from build123d import *

# Parameters (mm, degrees)
F0_W     = 25.4
F0_H     = 50.8
F0_W_2   = 19.05
F0_H_2   = 44.45
F1_DEPTH = 228.6
F2_W     = 25.4
F2_H     = 457.2
F2_R     = 2.5527
F3_DEPTH = 50.801


with BuildPart() as f1:
    # F0 (on Front) → F1 (new body, symmetric)
    with BuildSketch(Plane.XZ):
        Rectangle(F0_W, F0_H)
        Rectangle(F0_W_2, F0_H_2, mode=Mode.SUBTRACT)
    extrude(amount=F1_DEPTH, both=True)

    # F2 (on face) → F3 (intersect, through all)
    with BuildSketch(Plane.XY.offset(25.4)):
        Rectangle(F2_W, F2_H)
        with Locations((-1.224507, -215.9)):
            Circle(F2_R, mode=Mode.SUBTRACT)
        with Locations((-1.224507, -203.2)):
            Circle(F2_R, mode=Mode.SUBTRACT)
        with Locations((-1.224507, -190.5)):
            Circle(F2_R, mode=Mode.SUBTRACT)
        with Locations((-1.224507, -177.8)):
            Circle(F2_R, mode=Mode.SUBTRACT)
        with Locations((-1.224507, -165.1)):
            Circle(F2_R, mode=Mode.SUBTRACT)
        with Locations((-1.224507, -152.4)):
            Circle(F2_R, mode=Mode.SUBTRACT)
        with Locations((-1.224507, -139.7)):
            Circle(F2_R, mode=Mode.SUBTRACT)
        with Locations((-1.224507, -127)):
            Circle(F2_R, mode=Mode.SUBTRACT)
        with Locations((-1.224507, -114.3)):
            Circle(F2_R, mode=Mode.SUBTRACT)
        with Locations((-1.224507, -101.6)):
            Circle(F2_R, mode=Mode.SUBTRACT)
        with Locations((-1.224507, -88.9)):
            Circle(F2_R, mode=Mode.SUBTRACT)
        with Locations((-1.224507, -76.2)):
            Circle(F2_R, mode=Mode.SUBTRACT)
        with Locations((-1.224507, -63.5)):
            Circle(F2_R, mode=Mode.SUBTRACT)
        with Locations((-1.224507, -50.8)):
            Circle(F2_R, mode=Mode.SUBTRACT)
        with Locations((-1.224507, -38.1)):
            Circle(F2_R, mode=Mode.SUBTRACT)
        with Locations((-1.224507, -25.4)):
            Circle(F2_R, mode=Mode.SUBTRACT)
        with Locations((-1.224507, -12.7)):
            Circle(F2_R, mode=Mode.SUBTRACT)
        with Locations((-1.224507, 0)):
            Circle(F2_R, mode=Mode.SUBTRACT)
        with Locations((-1.224507, 12.7)):
            Circle(F2_R, mode=Mode.SUBTRACT)
        with Locations((-1.224507, 25.4)):
            Circle(F2_R, mode=Mode.SUBTRACT)
        with Locations((-1.224507, 38.1)):
            Circle(F2_R, mode=Mode.SUBTRACT)
        with Locations((-1.224507, 50.8)):
            Circle(F2_R, mode=Mode.SUBTRACT)
        with Locations((-1.224507, 63.5)):
            Circle(F2_R, mode=Mode.SUBTRACT)
        with Locations((-1.224507, 76.2)):
            Circle(F2_R, mode=Mode.SUBTRACT)
        with Locations((-1.224507, 88.9)):
            Circle(F2_R, mode=Mode.SUBTRACT)
        with Locations((-1.224507, 101.6)):
            Circle(F2_R, mode=Mode.SUBTRACT)
        with Locations((-1.224507, 114.3)):
            Circle(F2_R, mode=Mode.SUBTRACT)
        with Locations((-1.224507, 127)):
            Circle(F2_R, mode=Mode.SUBTRACT)
        with Locations((-1.224507, 139.7)):
            Circle(F2_R, mode=Mode.SUBTRACT)
        with Locations((-1.224507, 152.4)):
            Circle(F2_R, mode=Mode.SUBTRACT)
        with Locations((-1.224507, 165.1)):
            Circle(F2_R, mode=Mode.SUBTRACT)
        with Locations((-1.224507, 177.8)):
            Circle(F2_R, mode=Mode.SUBTRACT)
        with Locations((-1.224507, 190.5)):
            Circle(F2_R, mode=Mode.SUBTRACT)
        with Locations((-1.224507, 203.2)):
            Circle(F2_R, mode=Mode.SUBTRACT)
        with Locations((-1.224507, 215.9)):
            Circle(F2_R, mode=Mode.SUBTRACT)
    extrude(amount=-F3_DEPTH, mode=Mode.INTERSECT)


solid = f1.part
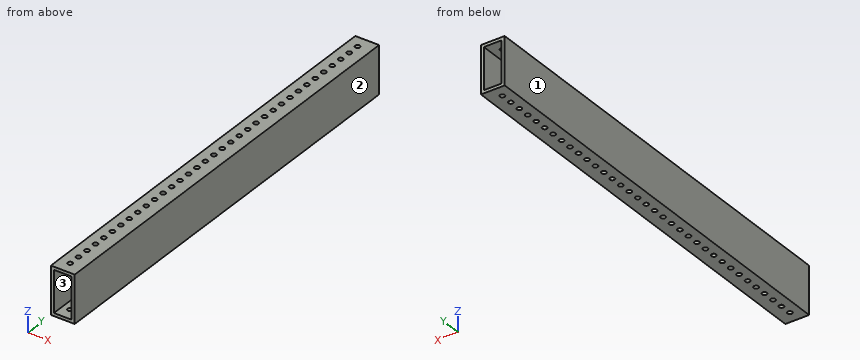
For this review, take the finished solid that the model builds, in its own axes (mm). Face numbers are marked on the shaded views. Coordinates: 2 decimals unless noted, no trailing zeros. Write each loop counter-clockwise with the first axis right and the second up, starting at its lowest first coordinate (ties: lowest second). Pieces come first, ordered by that corner, then holes. Notation, with made-up numbers: (3.5, 24.5) -> (59.5, 24.5) arc R28 ccw to (59.5, 53.5) -> close; hole circle Ø5 at (63.5, -33). An arc over 180 degrees is marked (long way). Write each question's results on one line, items separated by ' | '. Start each with the question number.
1) Consider section A-A (z = 13). Write out the cut boundary in (x, y) (3 decimals).
2) Insertion check: pin 1 (8 mm diameter, centred on x = -1.22, y = -114.3, fed in from -Z). The pin has a flat end and moves straight along its axis. Give the tip position at first contact, or say it passes through.
3) Wall thickness on L1, parallel to X at y = 114, z = 23; L2, parallel to Z at x = 3.75, y = -96 (3 decimals); L3, parallel to X at y = -1.5, z = -21 (3 decimals): over which ranges is each line inside the solid? List them lowest first. Write a range as [from, to].
4) The part is to be moulded in two halves that separate along X. For the marked faces 1, 2 and 3, say which applies: +X half, -X half, draft (parallel to the pull), parting line (faces both ways), or undercut.
Geometry says:
1) outline: (-12.7, -228.6) -> (-9.525, -228.6) -> (-9.525, 228.6) -> (-12.7, 228.6) -> close; (9.525, -228.6) -> (12.7, -228.6) -> (12.7, 228.6) -> (9.525, 228.6) -> close
2) pin 1: z = -25.4
3) L1: [-12.7, -3.76], [1.31, 12.7] | L2: [-25.4, -22.225], [22.225, 25.4] | L3: [-12.7, -9.525], [9.525, 12.7]
4) face 1: -X half | face 2: +X half | face 3: undercut
